```python
from build123d import *

# Parameters (mm, degrees)
SKETCH1_W                       = 101.6
SKETCH1_H                       = 101.6
BOSS_EXTRUDE1_DEPTH             = 3.81
M6X1_0_TAPPED_HOLE1_D           = 5
M6X1_0_TAPPED_HOLE1_CBORE_D     = 6
M6X1_0_TAPPED_HOLE1_CBORE_DEPTH = 3.048
SKETCH4_W                       = 101.6
SKETCH4_H                       = 62.23
BOSS_EXTRUDE2_DEPTH             = 9.525
BOSS_EXTRUDE3_DEPTH             = 9.525
BOSS_EXTRUDE4_DEPTH             = 9.525


with BuildPart() as part:
    # Sketch1 → Boss-Extrude1 (new body)
    with BuildSketch(Plane.XY):
        with Locations((-50.8, 50.8)):
            Rectangle(SKETCH1_W, SKETCH1_H)
    extrude(amount=BOSS_EXTRUDE1_DEPTH)

    # M6x1.0 Tapped Hole1 (through all)
    with Locations(Plane(origin=(-50.8, -38.1, 0), x_dir=(-1, 0, 0), z_dir=(0, 0, -1))):
        with Locations((-29.14300736, 61.964884424), (30.859893074, 61.964884424)):
            CounterBoreHole(M6X1_0_TAPPED_HOLE1_D / 2, M6X1_0_TAPPED_HOLE1_CBORE_D / 2, M6X1_0_TAPPED_HOLE1_CBORE_DEPTH)

    # Sketch4 → Boss-Extrude2 (add)
    with BuildSketch(Plane(origin=(0, 0, 0), x_dir=(-1, 0, 0), z_dir=(0, 0, -1))):
        with Locations((50.8, 70.485)):
            Rectangle(SKETCH4_W, SKETCH4_H)
    extrude(amount=BOSS_EXTRUDE2_DEPTH)

    # Sketch5 → Boss-Extrude3 (add)
    with BuildSketch(Plane(origin=(0, 0, 0), x_dir=(0, 0, -1), z_dir=(1, 0, 0))):
        Polygon((9.525, 101.6), (15.875, 101.6), (35.534233385, 50.8), (35.534233385, 25.4), (14.2748, 25.4), (14.2748, 39.37), (9.525, 39.37), align=None)
    extrude(amount=-BOSS_EXTRUDE3_DEPTH)

    # Sketch6 → Boss-Extrude4 (add)
    with BuildSketch(Plane.ZY.offset(101.6)):
        Polygon((-9.525, 39.37), (-9.525, 101.6), (-15.875, 101.6), (-35.534233385, 50.8), (-35.534233385, 25.4), (-14.2748, 25.4), (-14.2748, 39.37), align=None)
    extrude(amount=-BOSS_EXTRUDE4_DEPTH)


solid = part.part
```
CAD build for the part. Positions are in the model's coordinates, mm. A direction names the side the tool comes from. Round coordinates to 2 decimals unless told otherwise and drop trailing zeros. Order: outer loops, then holes, each group sorted by start corner. A loop starts at its lowest first (then second) coordinate and runs counter-clockwise, first axis right, second up.
Item 1: Mould opens along Z. For faces 6 (the face through (-52, 39.37, -6)), 7 (the face through (-9.525, 56, -20)), 8 (the face through (-20, 26, 3.048)) say: pulls with the +Z half, pulls with the -Z half, needs draft (parallel to the pull), parting line crosses it, or undercut.
Item 2: Saw through at B-B on z = -22. Write the cut outline in (x, y) (3 decimals), then the cut area to 3 significant figures.
Item 3: Probe line 1 along X through (y, z) = (57.5, -31) (3 decimals); line 2 along Z through (x, y) = (-36.5, 84) (3 decimals); line 3 along Y through (x, z) = (-8.5, -9.5). List the from-to ranges inside material, lowest first.
Item 4: Saw through at C-C on y = 42. Write the cut outline in (x, z) (3 decimals), then the cut area to 3 significant figures.
Item 5: Saw through at A-A on y = 31. Write the cut outline in (x, z) (3 decimals).
Item 6: Pin check, flat tips, straight feed: pin 1 (4 mm diameter, centred on x = -87.5, y = 25, fed in from -Z); pin 2 (7.5 mm diameter, centred on x = -5, z = -27, fed in from -Y); pin 3 (2 mm diameter, centred on x = -27.5, y = 44.5, fed in from -Z) (3 decimals). Stop position of each tip, or through.
Item 7: Tool access for faces 1 (the face through (-96.904, 76.556, -25.567)), 2 (the face through (-5, 32, -14.275)), 3 (the face through (-83.04, 21.2, 1.5)), 4 (the face through (-97, 25.4, -25)), 5 (the face through (-50, 71, -9.525)): list every direction of +Z, -Z, +X, -X, +Y, -Y with a clear straight run to the whole face (end or side of a thin tool).
Item 8: Saw through at D-D on x = -28. Write the cut outline in (y, z) (3 decimals), then the cut area to 3 significant figures.
Reported:
1. face 6: undercut
1. face 7: needs draft
1. face 8: pulls with the -Z half
2. outline: (-101.6, 25.4) - (-92.075, 25.4) - (-92.075, 85.773) - (-101.6, 85.773) - close; (-9.525, 25.4) - (0, 25.4) - (0, 85.773) - (-9.525, 85.773) - close
2. area: 1,150 mm2
3. line 1: x = -101.6 to -92.075, -9.525 to 0
3. line 2: z = -9.525 to 3.81
3. line 3: y = 39.37 to 101.6
4. outline: (-101.6, -35.534) - (-92.075, -35.534) - (-92.075, -9.525) - (-9.525, -9.525) - (-9.525, -35.534) - (0, -35.534) - (0, 3.81) - (-101.6, 3.81) - close
4. area: 1,850 mm2
5. outline: (-101.6, -35.534) - (-92.075, -35.534) - (-92.075, -14.275) - (-101.6, -14.275) - close; (-101.6, 0) - (0, 0) - (0, 3.81) - (-101.6, 3.81) - close; (-9.525, -35.534) - (0, -35.534) - (0, -14.275) - (-9.525, -14.275) - close
6. pin 1: stops at z = 0
6. pin 2: stops at y = 25.4
6. pin 3: stops at z = -9.525
7. face 1: -Z, +X, -X, +Y
7. face 2: +X, -X, -Y
7. face 3: -Z
7. face 4: -Z, +X, -X, -Y
7. face 5: -Z, +Y, -Y
8. outline: (0, 0) - (39.37, 0) - (39.37, -9.525) - (101.6, -9.525) - (101.6, 3.81) - (0, 3.81) - close
8. area: 980 mm2
